from build123d import *

# Parameters (mm, degrees)
SKETCH1_R           = 2.5
BOSS_EXTRUDE1_DEPTH = 5


with BuildPart() as part:
    # Sketch1 → Boss-Extrude1 (new body)
    with BuildSketch(Plane.XY):
        with BuildLine():
            Line((-59.996652166, 19.634073567), (-104.996652166, 19.634073567))
            ThreePointArc((-104.996652166, 19.634073567), (-109.996652166, 24.634073567), (-104.996652166, 29.634073567))
            Line((-104.996652166, 29.634073567), (-59.996652166, 29.634073567))
            ThreePointArc((-59.996652166, 29.634073567), (-54.996652166, 24.634073567), (-59.996652166, 19.634073567))
        make_face()
        with Locations((-59.996652166, 24.634073567)):
            Circle(SKETCH1_R, mode=Mode.SUBTRACT)
        with Locations((-104.996652166, 24.634073567)):
            Circle(SKETCH1_R, mode=Mode.SUBTRACT)
    extrude(amount=-BOSS_EXTRUDE1_DEPTH)


solid = part.part
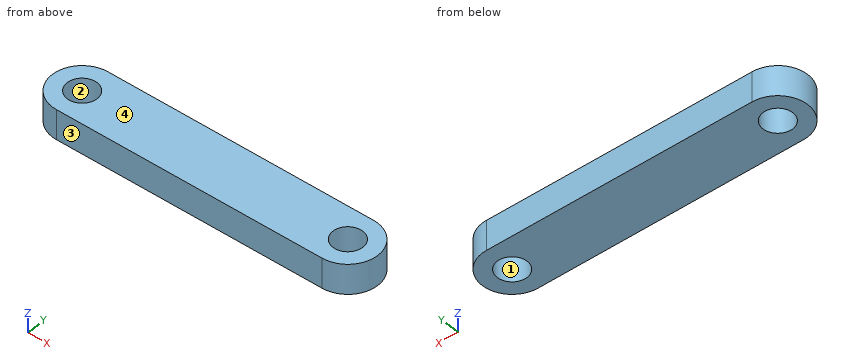
Here's how the part is built. I have some questions about the finished solid (model axes, mm). Face numbers are marked on the shaded views. Coordinates: 2 decimals unless noted, no trailing zeros. Loops run counter-clockwise (first coordinate to the right, second up) from the corner with the lowest first, then second, coordinate; pieces in that order, holes last. Notation, with made-up numbers: (-10, -22) -> (48, -22) arc R33 ccw to (48, 7) -> close; hole circle Ø8 at (-22, 41.25). An arc over 180 degrees is marked (long way). Use one line per item in the form item = value. Start each with the question number.
(1) If we section it at C-C (y = 26.25): Please give me the cut outline in (x, z), then the cut area to 3 significant figures.
(2) Will this pin go through, and if not, where does the flat tip stop? pin 1 (1.5 mm diameter, centred on x = -98, y = 23, fed in from +Z).
(3) If we section it at A-A (y = 23.25): Please give me the cut outline in (x, z).
(4) Please list where these lines run through material, in increasing order: line 1 along X through (y, z) = (24.75, -2.5); line 2 along X through (y, z) = (22.75, -0.25); line 3 along Y through (x, z) = (-61, -0.7).
(5) If we section it at D-D (z = -4.3): Please give me the cut outline in (x, y).
(6) If we section it at B-B (x = -62): Please give me the cut outline in (y, z).
(7) We'd pull the mould along Y, two halves only. Please class the marked faces 1, 2, 3 and 4: pulls with the +Y half, pulls with the -Y half, needs draft (parallel to the pull), parting line crosses it, or undercut.
Verdict:
q1.outline = (-109.73, -5) -> (-106.9, -5) -> (-106.9, 0) -> (-109.73, 0) -> close; (-103.09, -5) -> (-61.9, -5) -> (-61.9, 0) -> (-103.09, 0) -> close; (-58.09, -5) -> (-55.26, -5) -> (-55.26, 0) -> (-58.09, 0) -> close
q1.area = 234 mm²
q2.pin_1 = 0
q3.outline = (-109.8, -5) -> (-107.08, -5) -> (-107.08, 0) -> (-109.8, 0) -> close; (-102.91, -5) -> (-62.08, -5) -> (-62.08, 0) -> (-102.91, 0) -> close; (-57.91, -5) -> (-55.19, -5) -> (-55.19, 0) -> (-57.91, 0) -> close
q4.line_1 = -110 to -107.49, -102.5 to -62.49, -57.5 to -55
q4.line_2 = -109.63 to -106.64, -103.35 to -61.64, -58.35 to -55.37
q4.line_3 = 19.63 to 22.34, 26.92 to 29.63
q5.outline = (-105, 19.63) -> (-60, 19.63) arc R5 ccw to (-60, 29.63) -> (-105, 29.63) arc R5 ccw to start; hole circle Ø5 at (-105, 24.63); hole circle Ø5 at (-60, 24.63)
q6.outline = (19.63, -5) -> (23.14, -5) -> (23.14, 0) -> (19.63, 0) -> close; (26.13, -5) -> (29.63, -5) -> (29.63, 0) -> (26.13, 0) -> close
q7.face_1 = undercut
q7.face_2 = undercut
q7.face_3 = pulls with the -Y half
q7.face_4 = needs draft
